```python
from build123d import *

# Parameters (mm, degrees)
SKETCH1_W           = 150
SKETCH1_H           = 150
BOSS_EXTRUDE1_DEPTH = 5
SKETCH2_R           = 1.75
CUT_EXTRUDE1_DEPTH  = 213.190951739


with BuildPart() as part:
    # Sketch1 → Boss-Extrude1 (new body)
    with BuildSketch(Plane.XY):
        with Locations((75, 75)):
            Rectangle(SKETCH1_W, SKETCH1_H)
    extrude(amount=BOSS_EXTRUDE1_DEPTH)

    # Sketch2 → Cut-Extrude1 (cut, through all)
    with BuildSketch(Plane.XY.offset(5)):
        with Locations((73.960018565, 84)):
            Circle(SKETCH2_R)
        with Locations((73.960018565, 146)):
            Circle(SKETCH2_R)
        with Locations((135.960018565, 146)):
            Circle(SKETCH2_R)
        with Locations((135.960018565, 84)):
            Circle(SKETCH2_R)
        Polygon((77.960018565, 150), (131.960018565, 150), (131.960018565, 142), (139.960018565, 142), (139.960018565, 88), (131.960018565, 88), (131.960018565, 80), (77.960018565, 80), (77.960018565, 88), (69.960018565, 88), (69.960018565, 142), (77.960018565, 142), align=None)
    extrude(amount=-CUT_EXTRUDE1_DEPTH, mode=Mode.SUBTRACT)


solid = part.part
```
Geometry check sheet. Reference: the model listing, model coordinates, mm. A direction names the side the tool comes from. Round coordinates to 2 decimals unless told otherwise and drop trailing zeros. Loops run counter-clockwise (first coordinate to the right, second up) from the corner with the lowest first, then second, coordinate; pieces in that order, holes last. Notation, with made-up numbers: M -20,17.5 L 4,17.5 A26 cw 4,32.5 Z; hole C 36.25,31.25 d10. An arc over 180 degrees is marked long. Return JSON: item names as keys, results as strings. Group by question number.
(1) Section check A-A, the plane z = 3.8. Enter the section's corners in (x, y).
(2) Scan lines: line 1 along X through (y, z) = (146, 2.3); line 2 along X through (y, z) = (87, 4.1); line 3 along X through (y, z) = (111, 1.9). Record each from-to range of solid material in increasing order. Write a range as [from, to].
(3) Section check B-B, the plane y = 146. Enter the section's corners in (x, z).
(4) Section check C-C, the plane x = 116.5. Enter the section's corners in (y, z), and give its area (3 significant figures).
(5) Set-up check for faces 1 (the face through (77.96, 84, 3)), 2 (the face through (74, 59, 0)), 3 (the face through (139.96, 115, 3)): record each of +Z, -Z, +X, -X, +Y, -Y from which the full face is reachable in a straight line by a thin tool's end or side.
(6) Mould release check, pull along X, two halves, no side actions. Record for faces 4 (the face through (137.629, 84.526, 2.535)), 5 (the face through (141, 150, 2)), 6 (the face through (0, 74, 2)): pulls with the +X half, pulls with the -X half, needs draft (parallel to the pull), parting line crosses it, or undercut.
(7) Go/stop test with flat-tipped pins: pin 1 (8 mm diameter, centred on x = 18, y = 19.5, fed in from -Z); pin 2 (1.5 mm diameter, centred on x = 104.5, z = 2, fed in from +Y). Record where each tip stops, or that it passes through.
Data:
{
 "1": {"outline": "M 0,0 L 150,0 L 150,150 L 131.96,150 L 131.96,142 L 139.96,142 L 139.96,88 L 131.96,88 L 131.96,80 L 77.96,80 L 77.96,88 L 69.96,88 L 69.96,142 L 77.96,142 L 77.96,150 L 0,150 Z; hole C 73.96,84 d3.5; hole C 73.96,146 d3.5; hole C 135.96,84 d3.5; hole C 135.96,146 d3.5"},
 "2": {"line 1": "[0, 72.21], [75.71, 77.96], [131.96, 134.21], [137.71, 150]", "line 2": "[0, 77.96], [131.96, 150]", "line 3": "[0, 69.96], [139.96, 150]"},
 "3": {"outline": "M 0,0 L 72.21,0 L 72.21,5 L 0,5 Z; M 75.71,0 L 77.96,0 L 77.96,5 L 75.71,5 Z; M 131.96,0 L 134.21,0 L 134.21,5 L 131.96,5 Z; M 137.71,0 L 150,0 L 150,5 L 137.71,5 Z"},
 "4": {"outline": "M 0,0 L 80,0 L 80,5 L 0,5 Z", "area": "400 mm²"},
 "5": {"face 1": "+Z, -Z, +Y", "face 2": "-Z, +X, -X, +Y, -Y", "face 3": "+Z, -Z"},
 "6": {"face 4": "undercut", "face 5": "needs draft", "face 6": "pulls with the -X half"},
 "7": {"pin 1": "z = 0", "pin 2": "y = 80"}
}
